Input: part model. Units: mm. Frame: model coordinates. Face numbers are marked on the shaded views. A direction names the side the tool comes from. Round coordinates to 2 decimals unless told otherwise and drop trailing zeros. Write each loop counter-clockwise with the first axis right and the second up, starting at its lowest first coordinate (ties: lowest second). Pieces come first, ordered by that corner, then holes. Notation, with made-up numbers: (18, 19.25) - (68, 19.25) arc R26 cw to (68, 44.25) - close; hole circle Ø2 at (42, -39.5). An arc over 180 degrees is marked (long way). One line per item, written item: value. Start each with the question number.
```python
from build123d import *

# Parameters (mm, degrees)
REVOLVE_1_ANGLE          = 40
SKETCH_3_W               = 5.2
SKETCH_3_H               = 5.2
CUT_EXTRUDE_1_DEPTH      = 7
CUT_EXTRUDE_2_DEPTH      = 94.967026614
CUT_EXTRUDE_2_DEPTH_BACK = 94.967026614
SKETCH_5_R               = 1.5
CUT_EXTRUDE_START        = -2
SKETCH_6_R               = 3
CUT_EXTRUDE_3_DEPTH      = 93.938324905
SKETCH_12_R              = 1.5
CUT_EXTRUDE_5_DEPTH      = 54.141615619
CUT_EXTRUDE_6_DEPTH      = 5
PATTERN_CIRCULAR_1_COUNT = 4
PATTERN_CIRCULAR_1_ANGLE = 15
F_1_THE_OTHER_WAY_COUNT  = 4
F_1_THE_OTHER_WAY_ANGLE  = 15
SKETCH_9_W               = 1.8
SKETCH_9_H               = 4.8
SKETCH_9_H_2             = 2.8
EXTRUDE_2_DEPTH          = 3
SKETCH_10_W              = 52.448370613
SKETCH_10_H              = 39.953744926
CUT_EXTRUDE_4_DEPTH      = 149.179341739
SKETCH_11_W              = 14
SKETCH_11_H              = 30
EXTRUDE_3_DEPTH          = 5
FILLET_1_R               = 5


# Read off the part's stored shape, not the designer's step: 旋转1
with BuildPart() as part:
    # 旋转1 outline → 旋转1 (revolve)
    with BuildSketch(Plane(origin=(0, 0, 0), x_dir=(0.3420201433256701, 0, -0.9396926207859079), z_dir=(0.9396926207859079, 0, 0.3420201433256701))):
        Polygon((134, 5), (125, 5), (125, -5), (134, -5), (134, -7.5), (136.5, -10), (139, -7.5), (139, 7.5), (136.5, 10), (134, 7.5), align=None)
    revolve(axis=Axis((0, 0, 0), (0, 1, 0)), revolution_arc=REVOLVE_1_ANGLE)

    # 草图3 → 切除-拉伸1 (cut)
    with BuildSketch(Plane(origin=(0, 0, 0), x_dir=(0.34202014332566943, 0, -0.9396926207859081), z_dir=(0.9396926207859081, 0, 0.34202014332566943))):
        with Locations((132, 0)):
            Rectangle(SKETCH_3_W, SKETCH_3_H)
    extrude(amount=-CUT_EXTRUDE_1_DEPTH, mode=Mode.SUBTRACT)

    # 草图5 → 切除-拉伸2 (cut, two sides: drawn at the far end of the back side and taken through both)
    with BuildSketch(Plane(origin=(44.257406546, 0, -121.59622513), x_dir=(-0.9396926207859081, 0, -0.3420201433256695), z_dir=(0.3420201433256695, 0, -0.9396926207859081)).offset(-CUT_EXTRUDE_2_DEPTH_BACK)):
        with Locations((3.5, 0)):
            Circle(SKETCH_5_R)
    extrude(amount=CUT_EXTRUDE_2_DEPTH + CUT_EXTRUDE_2_DEPTH_BACK, mode=Mode.SUBTRACT)

    # 草图6 → 切除-拉伸3 (cut, through all)
    with BuildSketch(Plane(origin=(46.035911292, 0, -126.482626758), x_dir=(0.9396926207859081, 0, 0.3420201433256695), z_dir=(-0.3420201433256695, 0, 0.9396926207859081)).offset(CUT_EXTRUDE_START)):
        with Locations((-3.5, 0)):
            Circle(SKETCH_6_R)
    extrude(amount=-CUT_EXTRUDE_3_DEPTH, mode=Mode.SUBTRACT)

    # 草图12 → 切除-拉伸5 (cut, through all)
    with BuildSketch(Plane(origin=(0, 0, -139), x_dir=(-1, 0, 0), z_dir=(0, 0, -1))):
        Circle(SKETCH_12_R)
    cut_extrude_5 = extrude(amount=-CUT_EXTRUDE_5_DEPTH, mode=Mode.SUBTRACT)

    # 草图13 → 切除-拉伸6 (cut)
    with BuildSketch(Plane(origin=(0, 0, -139), x_dir=(-1, 0, 0), z_dir=(0, 0, -1))):
        Polygon((0, -3.175426481), (2.75, -1.58771324), (2.75, 1.58771324), (0, 3.175426481), (-2.75, 1.58771324), (-2.75, -1.58771324), align=None)
    cut_extrude_6 = extrude(amount=-CUT_EXTRUDE_6_DEPTH, mode=Mode.SUBTRACT)

    # 阵列(圆周)1: 切除-拉伸5, 切除-拉伸6 ×4 about axis
    pattern_circular_1_axis = Axis((0, 0, 0), (0, 1, 0))
    add([cut_extrude_5.rotate(pattern_circular_1_axis, i * PATTERN_CIRCULAR_1_ANGLE / (PATTERN_CIRCULAR_1_COUNT - 1)) for i in range(1, PATTERN_CIRCULAR_1_COUNT)], mode=Mode.SUBTRACT)
    add([cut_extrude_6.rotate(pattern_circular_1_axis, i * PATTERN_CIRCULAR_1_ANGLE / (PATTERN_CIRCULAR_1_COUNT - 1)) for i in range(1, PATTERN_CIRCULAR_1_COUNT)], mode=Mode.SUBTRACT)

    # 1 the other way: 切除-拉伸5, 切除-拉伸6 ×4 about axis
    f_1_the_other_way_axis = Axis((0, 0, 0), (0, -1, 0))
    add([cut_extrude_5.rotate(f_1_the_other_way_axis, i * F_1_THE_OTHER_WAY_ANGLE / (F_1_THE_OTHER_WAY_COUNT - 1)) for i in range(1, F_1_THE_OTHER_WAY_COUNT)], mode=Mode.SUBTRACT)
    add([cut_extrude_6.rotate(f_1_the_other_way_axis, i * F_1_THE_OTHER_WAY_ANGLE / (F_1_THE_OTHER_WAY_COUNT - 1)) for i in range(1, F_1_THE_OTHER_WAY_COUNT)], mode=Mode.SUBTRACT)

    # 草图9 → 凸台-拉伸2 (add)
    with BuildSketch(Plane(origin=(0, 0, 0), x_dir=(0.34202014332566943, 0, -0.9396926207859082), z_dir=(0.9396926207859082, 0, 0.34202014332566943))):
        with Locations((138.1, 0)):
            Rectangle(SKETCH_9_W, SKETCH_9_H)
        with Locations((125.9, 3.6)):
            Rectangle(SKETCH_9_W, SKETCH_9_H_2)
        with Locations((125.9, -3.6)):
            Rectangle(SKETCH_9_W, SKETCH_9_H_2)
    extrude(amount=EXTRUDE_2_DEPTH)

    # 草图10 → 切除-拉伸4 (cut, through all)
    with BuildSketch(Plane(origin=(0, 0, 0), x_dir=(0, -1, 0), z_dir=(0.9990482215818578, 0, -0.04361938736533606))):
        with Locations((1.816079314, 125.001454628)):
            Rectangle(SKETCH_10_W, SKETCH_10_H)
    extrude(amount=-CUT_EXTRUDE_4_DEPTH, mode=Mode.SUBTRACT)

    # 草图11 → 凸台-拉伸3 (add)
    with BuildSketch(Plane(origin=(0, 0, 0), x_dir=(0.043619387365336076, 0, 0.9990482215818578), z_dir=(-0.9990482215818577, 0, 0.04361938736533607))):
        with Locations((-132, 0)):
            Rectangle(SKETCH_11_W, SKETCH_11_H)
    extrude(amount=EXTRUDE_3_DEPTH)

    # 圆角1
    fillet_1_edges = [part.edges().sort_by_distance(p)[0] for p in [
        (-8.560715398, 15, -138.758654331),
        (-8.560715398, -15, -138.758654331),
        (-7.950043975, -15, -124.771979229),
        (-7.950043975, 15, -124.771979229),
    ]]
    fillet(fillet_1_edges, radius=FILLET_1_R)


solid = part.part
```
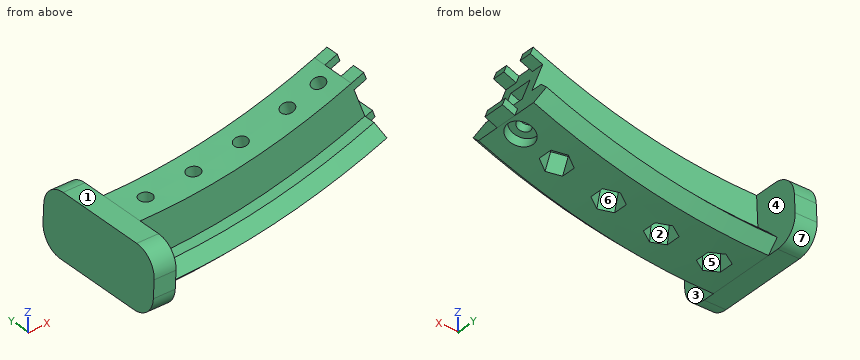
Q1. Material intervals for probe 1 along Y at (x, z) = (0, -127.25); probe 2 along X at (y, z) = (0, -131.75); probe 3 along Y at (x, z) = (4.5, -125.5), sorted ascending. Write a range as from..to.
Q2. Contact query for flat-ended pins moving along their axis: pin 1 Ø3 at (x, z) = (44.5, -118.5) entering from -Y; pin 2 Ø2 at (x, z) = (44.5, -117.5) entering from +Y; pin 3 Ø1.4 at (x, z) = (49, -129.5) entering from +Y; pin 4 Ø6 at (x, y) = (1, 1) entering from -Z. Output: stop coordinate, or through.
Q3. Pull-direction query (Z, two-part tool) for the marked faces 5, 6 and 7; classes: pulls with the +Z half, pulls with the -Z half, needs draft (parallel to the pull), parting line crosses it, or undercut.
Q4. Cut plane B-B, the plane y = 0. Count the separate pieces of the cut face and the enclosed holes in it, and give its area (3 significant figures).
Q5. Cut plane A-A, the plane y = -9. Output: boundary loops of the cut face in (x, z).
Q6. Access query for the marked faces 1, 2, 3 and 4. Directions: +Z, -Z, +X, -X, +Y, -Y. A direction counts if a zero-diameter tool reaches every point of the face in a straight line with its end or side. Return the directions, or none.
A:
1. probe 1: y = -5..-1.5, 1.5..5
1. probe 2: x = -10.76..-1.5, 1.5..10.02, 13.03..21.71, 26.02..32.46, 38.15..41.04
1. probe 3: y = -5..5
2. pin 1: stops at y = -5
2. pin 2: stops at y = 5
2. pin 3: stops at y = 2.4
2. pin 4: stops at z = -139
3. face 5: needs draft
3. face 6: undercut
3. face 7: pulls with the -Z half
4. separate pieces: 7
4. enclosed holes: 0
4. area: 513 mm²
5. outline: (-11.06, -138.65) - (-6.06, -138.87) - (-6, -137.37) arc R137.5 ccw to (47.03, -129.21) - (46.34, -127.33) arc R135.5 cw to (-5.91, -135.37) - (-5.45, -124.88) - (-10.45, -124.66) - close
6. face 1: +Z, +Y, -Y
6. face 2: none
6. face 3: -Y
6. face 4: +Y
